from build123d import *

# Parameters (mm, degrees)
BOSS_EXTRUDE1_DEPTH = 2.5
BOSS_EXTRUDE2_DEPTH = 4.5
SKETCH3_W           = 0.753987371
SKETCH3_H           = 12.516496397
BOSS_EXTRUDE3_DEPTH = 2.5
BOSS_EXTRUDE4_DEPTH = 29.5


with BuildPart() as part:
    # Sketch1 → Boss-Extrude1 (new body)
    with BuildSketch(Plane(origin=(0, 0, 0), x_dir=(1, 0, 0), z_dir=(0, 1, 0))):
        with BuildLine():
            Line((23.5, -23.5), (-23.5, -23.5))
            Line((-23.5, -23.5), (-25.258661881, -23.5))
            ThreePointArc((-25.258661881, -23.5), (12.625889377, -32.106649116), (34.5, 0))
            ThreePointArc((34.5, 0), (-5.56461177, 34.04827596), (-32.704933093, -10.983503603))
            Line((-32.704933093, -10.983503603), (-23.5, -10.983503603))
            Line((-23.5, -10.983503603), (-23.5, 23.5))
            Line((-23.5, 23.5), (23.5, 23.5))
            Line((23.5, 23.5), (23.5, -10.983503603))
            Line((23.5, -10.983503603), (31.93538088, -10.983503603))
            ThreePointArc((31.93538088, -10.983503603), (28.783275467, -17.66434139), (24.253987371, -23.5))
            Line((24.253987371, -23.5), (23.5, -23.5))
        make_face()
    extrude(amount=BOSS_EXTRUDE1_DEPTH)

    # Sketch2 → Boss-Extrude2 (add)
    with BuildSketch(Plane(origin=(0, 2.5, 0), x_dir=(1, 0, 0), z_dir=(0, 1, 0))):
        with BuildLine():
            Line((23.5, 23.5), (23.5, -10.983503603))
            Line((23.5, -10.983503603), (31.93538088, -10.983503603))
            ThreePointArc((31.93538088, -10.983503603), (28.783275467, -17.66434139), (24.253987371, -23.5))
            Line((24.253987371, -23.5), (15.688360219, -23.5))
            Line((15.688360219, -23.5), (15.688360219, -30.726622881))
            ThreePointArc((15.688360219, -30.726622881), (13.032214999, 31.943878478), (-32.704933093, -10.983503603))
            Line((-32.704933093, -10.983503603), (-23.5, -10.983503603))
            Line((-23.5, -10.983503603), (-23.5, 23.5))
            Line((-23.5, 23.5), (23.5, 23.5))
        make_face()
        with BuildLine():
            Line((11.957302625, -23.5), (-25.258661881, -23.5))
            ThreePointArc((-25.258661881, -23.5), (-7.991464927, -33.561681846), (11.957302625, -32.361596282))
            Line((11.957302625, -32.361596282), (11.957302625, -23.5))
        make_face()
    extrude(amount=BOSS_EXTRUDE2_DEPTH)

    # Sketch3 → Boss-Extrude3 (add)
    with BuildSketch(Plane(origin=(0, 7, 0), x_dir=(1, 0, 0), z_dir=(0, 1, 0))):
        with BuildLine():
            Line((-23.5, -23.5), (-23.5, -10.983503603))
            Line((-23.5, -10.983503603), (-32.704933093, -10.983503603))
            ThreePointArc((-32.704933093, -10.983503603), (-14.895360155, -31.118776419), (11.957302625, -32.361596282))
            Line((11.957302625, -32.361596282), (11.957302625, -23.5))
            Line((11.957302625, -23.5), (-23.5, -23.5))
        make_face()
        with Locations((23.876993686, -17.241751802)):
            Rectangle(SKETCH3_W, SKETCH3_H)
        with BuildLine():
            ThreePointArc((31.93538088, -10.983503603), (28.783275467, -17.66434139), (24.253987371, -23.5))
            Line((24.253987371, -23.5), (15.688360219, -23.5))
            Line((15.688360219, -23.5), (15.688360219, -30.726622881))
            ThreePointArc((15.688360219, -30.726622881), (13.032214999, 31.943878478), (-32.704933093, -10.983503603))
            Line((-32.704933093, -10.983503603), (-23.5, -10.983503603))
            Line((-23.5, -10.983503603), (-23.5, 23.5))
            Line((-23.5, 23.5), (23.5, 23.5))
            Line((23.5, 23.5), (23.5, -10.983503603))
            Line((23.5, -10.983503603), (31.93538088, -10.983503603))
        make_face()
    extrude(amount=BOSS_EXTRUDE3_DEPTH)

    # Sketch4 → Boss-Extrude4 (add)
    # profile 1 of 2: a face of its own
    with BuildSketch(Plane(origin=(0, 9.5, 0), x_dir=(1, 0, 0), z_dir=(0, 1, 0))):
        with BuildLine():
            Line((11.957302625, -23.5), (-23.5, -23.5))
            Line((-23.5, -23.5), (-23.5, 23.5))
            Line((-23.5, 23.5), (23.5, 23.5))
            Line((23.5, 23.5), (23.5, -23.5))
            Line((23.5, -23.5), (15.688360219, -23.5))
            Line((15.688360219, -23.5), (15.688360219, -30.726622881))
            ThreePointArc((15.688360219, -30.726622881), (29.423616599, -18.013905357), (34.5, 0))
            ThreePointArc((34.5, 0), (-28.308805525, 19.71957225), (11.957302625, -32.361596282))
            Line((11.957302625, -32.361596282), (11.957302625, -23.5))
        make_face()
        with BuildLine():
            ThreePointArc((31.93538088, -10.983503603), (28.783275467, -17.66434139), (24.253987371, -23.5))
            Line((24.253987371, -23.5), (24.253987371, -10.983503603))
            Line((24.253987371, -10.983503603), (24.253987371, 23.5))
            ThreePointArc((24.253987371, 23.5), (27.378747533, 19.771446252), (29.93538088, 15.632622139))
            Line((29.93538088, 15.632622139), (29.93538088, -10.983503603))
            Line((29.93538088, -10.983503603), (31.93538088, -10.983503603))
        make_face(mode=Mode.SUBTRACT)
    # profile 2 of 2: a face of its own
    with BuildSketch(Plane(origin=(0, 9.5, 0), x_dir=(1, 0, 0), z_dir=(0, 1, 0))):
        with BuildLine():
            Line((15.688360219, -23.5), (11.957302625, -23.5))
            Line((11.957302625, -23.5), (11.957302625, -32.361596282))
            ThreePointArc((11.957302625, -32.361596282), (13.846983535, -31.599225417), (15.688360219, -30.726622881))
            Line((15.688360219, -30.726622881), (15.688360219, -23.5))
        make_face()
    extrude(amount=BOSS_EXTRUDE4_DEPTH)


solid = part.part
Here's how the part is built. I have some questions about the finished solid (model axes, mm). A direction names the side the tool comes from. Round coordinates to 2 decimals unless told otherwise and drop trailing zeros. Order: outer loops, then holes, each group sorted by start corner. A loop starts at its lowest first (then second) coordinate and runs counter-clockwise, first axis right, second up. Notation, with made-up numbers: (51, -6.75) -> (57, -6.75) arc R19 cw to (57, 5.25) -> close; hole circle Ø8 at (7, 40.25). An arc over 180 degrees is marked (long way). Return JSON: item names as keys, results as strings.
Q1. If we section it at C-C on z = -2: List the corners of the cut face in (x, y) for me.
Filled sheet:
{"outline": "(-34.44, 0) -> (-23.5, 0) -> (-23.5, 39) -> (-34.44, 39) -> close; (23.5, 0) -> (34.44, 0) -> (34.44, 39) -> (29.94, 39) -> (29.94, 9.5) -> (24.25, 9.5) -> (24.25, 39) -> (23.5, 39) -> close"}
Q2. If we section it at A-A on y = 5.5: List the corners of the cut face in (x, z) for me.
Filled sheet:
{"outline": "(-32.7, 10.98) arc R34.5 ccw (long way) to (15.69, 30.73) -> (15.69, 23.5) -> (24.25, 23.5) arc R33.77 cw to (31.94, 10.98) -> (23.5, 10.98) -> (23.5, -23.5) -> (-23.5, -23.5) -> (-23.5, 10.98) -> close; (-25.26, 23.5) -> (11.96, 23.5) -> (11.96, 32.36) arc R34.5 ccw to start"}
Q3. Which directions (+Z, -Z, +X, -X, +Y, -Y) give clear straight access to the entire face, cutting with the end or side of a thin tool? Please do faces 3 (the flat face through (23.5, 19, 0)), 4 (the flat face through (27, 9.5, -6)), 5 (the flat face through (14, 9.5, 28)).
Filled sheet:
{"face 3": "+Y, -Y", "face 4": "+Y", "face 5": "+Z"}
Q4. I need wall thicknesses on line 1 along X through (y, z) = (28.5, 6.5); line 2 along X through (y, z) = (33.5, 21); line 3 along Z through (x, y) = (-14.5, 24.5). Which ranges of each line are inside material? Lowest first, please. Write a range as from..to.
Filled sheet:
{"line 1": "x = -33.88..-23.5, 23.5..24.25, 29.94..33.88", "line 2": "x = -27.37..-23.5, 23.5..24.25, 26.45..27.37", "line 3": "z = -31.3..-23.5, 23.5..31.3"}
Q5. For pin 1 Ø8 at (y, z) = (15.5, 24.5) entering from +X; pin 2 Ø8 at (y, z) = (21, -2) entering from -X; pin 3 Ø3 at (x, z) = (-30, 18) entering from -Y; pin 4 Ø4 at (x, y) = (23, 15.5) entering from -Z, each with a flat end and sliding along its axis, tell me the tip position at first contact or that it passes through.
Filled sheet:
{"pin 1": "stops at x = 27.75", "pin 2": "stops at x = -34.5", "pin 3": "stops at y = 7", "pin 4": "stops at z = -27.37"}
Q6. If we section it at D-D on y = 17.5: List the corners of the cut face in (x, z) for me.
Filled sheet:
{"outline": "circle Ø69 at (0, 0); hole (-23.5, -23.5) -> (23.5, -23.5) -> (23.5, 23.5) -> (-23.5, 23.5) -> close; hole (24.25, -23.5) arc R33.77 ccw to (29.94, -15.63) -> (29.94, 10.98) -> (31.94, 10.98) arc R33.77 ccw to (24.25, 23.5) -> close"}
Q7. If we section it at B-B on x = 0: List the corners of the cut face in (y, z) for me, plus the area to 3 significant figures.
Filled sheet:
{"outline": "(0, -34.5) -> (39, -34.5) -> (39, -23.5) -> (0, -23.5) -> close; (0, 23.5) -> (39, 23.5) -> (39, 34.5) -> (0, 34.5) -> close", "area": "858 mm^2"}
Q8. If we mould it in two halves opening along Z, with no side actions, what happens to faces 1 (the flat face through (-28, 3, 10.984)), 2 (the flat face through (15.688, 6, 27))? For each: released by +Z, released by -Z, zero draft, split by the parting line, or undercut.
Filled sheet:
{"face 1": "undercut", "face 2": "zero draft"}
